Geometry check sheet. Reference: the model listing, model coordinates, mm. A direction names the side the tool comes from. Give positions to 0.01 mm unless a question says otherwise; leave off trailing zeros. Order: outer loops, then holes, each group sorted by start corner. A loop starts at its lowest first (then second) coordinate and runs counter-clockwise, first axis right, second up.
from build123d import *

# Parameters (mm, degrees)
EXTRUDE_1_DEPTH      = 15
EXTRUDE_7_DEPTH      = 15
EXTRUDE_7_DEPTH_BACK = 15
SKETCH_2_W           = 10
SKETCH_2_H           = 15


with BuildPart() as part:
    # 草图1 → 凸台-拉伸1 (new body)
    with BuildSketch(Plane(origin=(0, 0, 0), x_dir=(1, 0, 0), z_dir=(0, 1, 0))):
        Polygon((0, 0), (7, 0), (15, -6), (23, 0), (30, 0), (30, -28), (0, -28), align=None)
    extrude(amount=EXTRUDE_1_DEPTH)

    # 草图2 → 凸台-拉伸7 (add, two sides: drawn at the far end of the back side and taken through both)
    with BuildSketch(Plane(origin=(0, 15, 0), x_dir=(1, 0, 0), z_dir=(0, 1, 0)).offset(-EXTRUDE_7_DEPTH_BACK)):
        with Locations((30, -20.531171216)):
            Rectangle(SKETCH_2_W, SKETCH_2_H)
        with Locations((0, -20.5)):
            Rectangle(SKETCH_2_W, SKETCH_2_H)
    extrude(amount=EXTRUDE_7_DEPTH + EXTRUDE_7_DEPTH_BACK)


solid = part.part
Item 1: Gauge pin test, flat ends, axial feed: pin 1 (8.5 mm diameter, centred on x = 12.5, z = 18, fed in from +Y); pin 2 (12 mm diameter, centred on x = 17.5, y = 4.5, fed in from +Z); pin 3 (6.5 mm diameter, centred on y = 5.5, z = 8.5, fed in from +X). Record the tip position at first contact, or that the pin passes through.
Reported:
pin 1: stops at y = 15
pin 2: stops at z = 28
pin 3: stops at x = 30
Item 2: Scan lines: L1, parallel to X at y = 18.5, z = 26.5; L2, parallel to Y at x = 21, z = 24; L3, parallel to Z at x = 6, y = 9.75. Record each from-to range of solid material in increasing order.
Reported:
L1: x = -5 to 5, 25 to 35
L2: y = 0 to 15
L3: z = 0 to 28
Item 3: Sectioned sample at B-B (z = 13.5). Enter the section's corners in (x, y), and give its area (3 significant figures).
Reported:
outline: (-5, 0) - (35, 0) - (35, 30) - (25, 30) - (25, 15) - (5, 15) - (5, 30) - (-5, 30) - close
area: 900 mm2
Item 4: Draft check along X on faces 5 (the flat face through (19, 7, 3)), 6 (the flat face through (11, 7, 3)), 7 (the flat face through (3, 7, 0)), 8 (the flat face through (35, 15, 21)). Enter one of: released by +X, released by -X, zero draft, split by the parting line, or undercut.
Reported:
face 5: undercut
face 6: undercut
face 7: zero draft
face 8: released by +X
Item 5: Sectioned sample at A-A (y = 24). Enter the section's corners in (x, z).
Reported:
outline: (-5, 13) - (5, 13) - (5, 28) - (-5, 28) - close; (25, 13.03) - (35, 13.03) - (35, 28.03) - (25, 28.03) - close
Item 6: Set-up check for faces 1 (the flat face through (5, 22, 21)), 2 (the flat face through (0, 7, 7)), 3 (the flat face through (30, 7, 6)), 4 (the flat face through (30, 30, 20)): record each of +Z, -Z, +X, -X, +Y, -Y from which the full face is reachable in a straight line by a thin tool's end or side.
Reported:
face 1: +Z, -Z, +Y
face 2: -Z, -X, +Y, -Y
face 3: -Z, +X, +Y, -Y
face 4: +Z, -Z, +X, -X, +Y
Item 7: Sectioned sample at D-D (x = 27.5). Enter the section's corners in (y, z).
Reported:
outline: (0, 0) - (15, 0) - (15, 13.03) - (30, 13.03) - (30, 28.03) - (0, 28.03) - close
